Read the model definition and answer for the solid it produces. Units are mm, in the model's axes. A direction names the side the tool comes from. Give positions to 0.01 mm unless a question says otherwise; leave off trailing zeros. Order: outer loops, then holes, each group sorted by start corner. A loop starts at its lowest first (then second) coordinate and runs counter-clockwise, first axis right, second up. Notation, with made-up numbers: M -19,-32 L 6,-32 A25 ccw 6,-15 Z; hole C 37,-32 d5. An arc over 180 degrees is marked long. One line per item, written item: value.
from build123d import *

# Parameters (mm, degrees)
SKETCH1_W           = 437.35
SKETCH1_H           = 195
SKETCH1_R           = 4.1
SKETCH1_R_2         = 10
BOSS_EXTRUDE1_DEPTH = 6.35


with BuildPart() as part:
    # Sketch1 → Boss-Extrude1 (new body)
    with BuildSketch(Plane.XY):
        with Locations((-1.325, -19)):
            Rectangle(SKETCH1_W, SKETCH1_H)
        with Locations((-193.65, 58.5)):
            Circle(SKETCH1_R, mode=Mode.SUBTRACT)
        with Locations((-153.65, 58.5)):
            Circle(SKETCH1_R, mode=Mode.SUBTRACT)
        with Locations((-153.65, 18.5)):
            Circle(SKETCH1_R, mode=Mode.SUBTRACT)
        with Locations((-193.65, 18.5)):
            Circle(SKETCH1_R, mode=Mode.SUBTRACT)
        with Locations((-193.65, -56.5)):
            Circle(SKETCH1_R, mode=Mode.SUBTRACT)
        with Locations((-153.65, -56.5)):
            Circle(SKETCH1_R, mode=Mode.SUBTRACT)
        with Locations((-153.65, -96.5)):
            Circle(SKETCH1_R, mode=Mode.SUBTRACT)
        with Locations((-193.65, -96.5)):
            Circle(SKETCH1_R, mode=Mode.SUBTRACT)
        with Locations((157.35, -56.5)):
            Circle(SKETCH1_R, mode=Mode.SUBTRACT)
        with Locations((197.35, -56.5)):
            Circle(SKETCH1_R, mode=Mode.SUBTRACT)
        with Locations((197.35, -96.5)):
            Circle(SKETCH1_R, mode=Mode.SUBTRACT)
        with Locations((157.35, -96.5)):
            Circle(SKETCH1_R, mode=Mode.SUBTRACT)
        with Locations((157.35, 18.5)):
            Circle(SKETCH1_R, mode=Mode.SUBTRACT)
        with Locations((197.35, 18.5)):
            Circle(SKETCH1_R, mode=Mode.SUBTRACT)
        with Locations((197.35, 58.5)):
            Circle(SKETCH1_R, mode=Mode.SUBTRACT)
        with Locations((157.35, 58.5)):
            Circle(SKETCH1_R, mode=Mode.SUBTRACT)
        with Locations((-92.3, -96.5)):
            Circle(SKETCH1_R_2, mode=Mode.SUBTRACT)
        with Locations((-20, -96.5)):
            Circle(SKETCH1_R, mode=Mode.SUBTRACT)
        with Locations((20, -96.5)):
            Circle(SKETCH1_R, mode=Mode.SUBTRACT)
        with BuildLine():
            Line((-48.6, -44.5), (-48.6, -29.5))
            ThreePointArc((-48.6, -29.5), (-44.5, -25.4), (-40.4, -29.5))
            Line((-40.4, -29.5), (-40.4, -44.5))
            ThreePointArc((-40.4, -44.5), (-44.5, -48.6), (-48.6, -44.5))
        make_face(mode=Mode.SUBTRACT)
        with BuildLine():
            Line((-48.6, 44.5), (-48.6, 59.5))
            ThreePointArc((-48.6, 59.5), (-44.5, 63.6), (-40.4, 59.5))
            Line((-40.4, 59.5), (-40.4, 44.5))
            ThreePointArc((-40.4, 44.5), (-44.5, 40.4), (-48.6, 44.5))
        make_face(mode=Mode.SUBTRACT)
        with BuildLine():
            Line((40.4, 44.5), (40.4, 59.5))
            ThreePointArc((40.4, 59.5), (44.5, 63.6), (48.6, 59.5))
            Line((48.6, 59.5), (48.6, 44.5))
            ThreePointArc((48.6, 44.5), (44.5, 40.4), (40.4, 44.5))
        make_face(mode=Mode.SUBTRACT)
        with BuildLine():
            Line((40.4, -44.5), (40.4, -29.5))
            ThreePointArc((40.4, -29.5), (44.5, -25.4), (48.6, -29.5))
            Line((48.6, -29.5), (48.6, -44.5))
            ThreePointArc((48.6, -44.5), (44.5, -48.6), (40.4, -44.5))
        make_face(mode=Mode.SUBTRACT)
        with BuildLine():
            Line((-30, 0), (-30, 15))
            ThreePointArc((-30, 15), (0, 45), (30, 15))
            Line((30, 15), (30, 0))
            ThreePointArc((30, 0), (0, -30), (-30, 0))
        make_face(mode=Mode.SUBTRACT)
    extrude(amount=BOSS_EXTRUDE1_DEPTH)


solid = part.part
1) Find section A-A, the plane y = -96.5. Count the separate pieces of the cut face and the enclosed holes in it, plus the area to 3 significant figures.
Reported:
separate pieces: 8
enclosed holes: 0
area: 2,340 mm^2
2) Determine the mould class of faces 1 (the face through (-189.74, 19.73, 3.13)), 2 (the face through (-4, -39, 6.35)) for opening direction X: +X half, -X half, draft (parallel to the pull), parting line (faces both ways), or undercut.
Reported:
face 1: undercut
face 2: draft
3) Consider probe 1 along Y at (x, z) = (157.35, 2.25); probe 2 along X at (y, z) = (-26, 3.5); probe 3 along X at (y, z) = (4, 2.25). Determine where each line is inside the solid, lowest interval first.
Reported:
probe 1: y = -116.5 to -100.6, -92.4 to -60.6, -52.4 to 14.4, 22.6 to 54.4, 62.6 to 78.5
probe 2: x = -220 to -46.64, -42.36 to -14.97, 14.97 to 42.36, 46.64 to 217.35
probe 3: x = -220 to -30, 30 to 217.35
4) Find section D-D, the plane y = -13. Write down the section's boundary in (x, z).
Reported:
outline: M -220,0 L -27.04,0 L -27.04,6.35 L -220,6.35 Z; M 27.04,0 L 217.35,0 L 217.35,6.35 L 27.04,6.35 Z
5) Which of the six approach directions +Z, -Z, +X, -X, +Y, -Y give full straight-line access (tool end or side, diameter ignored) to faces 3 (the face through (-4, -39, 0)), 4 (the face through (0.66, -29.993, 3.131))?
Reported:
face 3: -Z, +X, -X, +Y, -Y
face 4: +Z, -Z
6) Find section C-C, the plane x = 8. Write down the section's boundary in (y, z), plus the area to 3 significant figures.
Reported:
outline: M -116.5,0 L -28.91,0 L -28.91,6.35 L -116.5,6.35 Z; M 43.91,0 L 78.5,0 L 78.5,6.35 L 43.91,6.35 Z
area: 776 mm^2
7) Find section B-B, the plane x = -153.65. Write down the section's boundary in (y, z).
Reported:
outline: M -116.5,0 L -100.6,0 L -100.6,6.35 L -116.5,6.35 Z; M -92.4,0 L -60.6,0 L -60.6,6.35 L -92.4,6.35 Z; M -52.4,0 L 14.4,0 L 14.4,6.35 L -52.4,6.35 Z; M 22.6,0 L 54.4,0 L 54.4,6.35 L 22.6,6.35 Z; M 62.6,0 L 78.5,0 L 78.5,6.35 L 62.6,6.35 Z
